Solid Edge part; units mm, degrees
sketch "Sketch1" plane through (0, 0, 0) normal (0, -1, 0) x (1, 0, 0)
  line L0 (40, 40) -> (-40, 40)
  line L1 (-40, 40) -> (-40, -40)
  line L2 (-40, -40) -> (40, -40)
  line L3 (40, -40) -> (40, 40)
  circle A0 centre (0, 0) radius 9
extrude "Extrusionsausprägung_23" add sketch "Sketch1" against normal blind 10
sketch "Sketch2" plane through (0, 0, 0) normal (0, -1, 0) x (1, 0, 0)
  circle A0 centre (-30, 30) radius 6.35
  circle A1 centre (30, 30) radius 6.35
  circle A2 centre (30, -30) radius 6.35
  circle A3 centre (-30, -30) radius 6.35
extrude "Extrusionsausschnitt_26" cut sketch "Sketch2" against normal blind 274
hole "Bohrung_9" at (16, 0, 16) direction (0, 1, 0) diameter 4 end up to next
hole "Hole1" at (16, 0, -16) direction (0, 1, 0) diameter 4 end up to next
hole "Hole2" at (-16, 0, -16) direction (0, 1, 0) diameter 4 end up to next
hole "Hole3" at (-16, 0, 16) direction (0, 1, 0) diameter 4 end up to next
sketch "Sketch3" plane through (0, 0, 0) normal (0, -1, 0) x (1, 0, 0)
  line L0 (9, 50) -> (-9, 50)
  line L1 (-9, 50) -> (-9, 0)
  line L2 (-9, 0) -> (9, 0)
  line L3 (9, 0) -> (9, 50)
extrude "Extrusionsausschnitt_27" cut sketch "Sketch3" against normal blind 138
sketch "Sketch4" plane through (0, 0, 0) normal (0, -1, 0) x (1, 0, 0)
  line L0 (-14, 12.5) -> (-30, 12.5)
  line L1 (-30, 12.5) -> (-30, -12.5)
  line L2 (-30, -12.5) -> (-14, -12.5)
  line L3 (-14, -12.5) -> (-14, 12.5)
extrude "Extrusionsausschnitt_28" cut sketch "Sketch4" against normal blind 67
fillet "Verrundung_16" radius 4 4 edges at (-30, 5, 12.5) (-14, 5, 12.5) (-30, 5, -12.5) (-14, 5, -12.5)
mirror "Mirror1" about plane through (0, 0, 0) normal (1, 0, 0) of "Extrusionsausschnitt_28", "Verrundung_16"
Could you check a few things on this model? Use its own coordinates, in mm. A direction names the side the tool comes from. Coordinates: 2 decimals unless noted, no trailing zeros. Order: outer loops, then holes, each group sorted by start corner. A loop starts at its lowest first (then second) coordinate and runs counter-clockwise, first axis right, second up. Notation, with made-up numbers: M 51.5,-34 L 97.5,-34 A27 cw 97.5,-9 Z; hole C 54.5,47 d6. An arc over 180 degrees is marked long. Use one line per item in the form item = value. Start each with the question number.
1. Suppose I cut it at A-A on z = -30. Write out the boundary of the cut face in (x, y), then the cut area to 3 significant figures.
2. Suppose I cut it at B-B on y = 2.75. Count the separate pieces of the cut face and the enclosed holes in it, then the cut area to 3 significant figures.
3. Please list where these lines run through material, in increasing order: line 1 (X direction, y = 3.25, z = 16); line 2 (X direction, y = 7.75, z = 4); line 3 (X direction, y = 3.5, z = 22).
4. Suppose I cut it at D-D on z = 16. Write out the boundary of the cut face in (x, y), then the cut area to 3 significant figures.
5. For pin 1 (3 mm diameter, centred on x = 16, z = -16, fed in from -Y), with a flat end and sliding along its axis, tell me the tip position at first contact or that it passes through.
6. Suppose I cut it at C-C on x = -20. Write out the boundary of the cut face in (y, z).
7. We'd pull the mould along Z, two halves only. Please class faces 1 (the flat face through (-40, 5, 1)), 2 (the flat face through (25, 5, 40)), 3 (the cylindrical face through (18, 5, -16)), 4 (the flat face through (-1, 5, -40)): +Z half, -Z half, draft (parallel to the pull), parting line (faces both ways), or undercut.
8. On a 3-axis mill with a long thin cutter (end or side, diameter ignored), from which of +Z, -Z, +X, -X, +Y, -Y can I reach the whole of each face in a straight line? I mean faces 5 (the flat face through (9.4, 0, 0.6)), 6 (the flat face through (30, 5, 0)), 7 (the flat face through (9, 5, 20)). Say none if no direction works.
Geometry says:
q1.outline = M -40,0 L -36.35,0 L -36.35,10 L -40,10 Z; M -23.65,0 L 23.65,0 L 23.65,10 L -23.65,10 Z; M 36.35,0 L 40,0 L 40,10 L 36.35,10 Z
q1.area = 546 mm^2
q2.separate_pieces = 1
q2.enclosed_holes = 10
q2.area = 4,220 mm^2
q3.line_1 = -40 to -18, -14 to -9, 9 to 14, 18 to 40
q3.line_2 = -40 to -30, -14 to -9, 9 to 14, 30 to 40
q3.line_3 = -40 to -9, 9 to 40
q4.outline = M -40,0 L -18,0 L -18,10 L -40,10 Z; M -14,0 L -9,0 L -9,10 L -14,10 Z; M 9,0 L 14,0 L 14,10 L 9,10 Z; M 18,0 L 40,0 L 40,10 L 18,10 Z
q4.area = 540 mm^2
q5.pin_1 = through
q6.outline = M 0,-40 L 10,-40 L 10,-12.5 L 0,-12.5 Z; M 0,12.5 L 10,12.5 L 10,40 L 0,40 Z
q7.face_1 = draft
q7.face_2 = +Z half
q7.face_3 = undercut
q7.face_4 = -Z half
q8.face_5 = +Z, -Z, +X, -X, -Y
q8.face_6 = +Y, -Y
q8.face_7 = +Z, +Y, -Y
